Read the model definition and answer for the solid it produces. Units are mm, in the model's axes. A direction names the side the tool comes from. Round coordinates to 2 decimals unless told otherwise and drop trailing zeros. Order: outer loops, then holes, each group sorted by start corner. A loop starts at its lowest first (then second) coordinate and runs counter-clockwise, first axis right, second up. Notation, with made-up numbers: (62, 19) - (70, 19) arc R13 cw to (70, 34) - close; hole circle Ø11 at (44.25, 77). An arc over 180 degrees is marked (long way). Answer as a JSON object with one key per item and string values. Group by question number.
Q1. A cutting plane is placed at D-D on y = 9.1. Determine the outline of the cut face in (x, z), and give its area (3 significant figures).
Q2. A cutting plane is placed at A-A on y = 16.8. Determine the outline of the cut face in (x, z), and give its area (3 significant figures).
Q3. Given pin 1 Ø6.5 at (y, z) = (15, 10.5) entering from -X; pin 2 Ø6 at (y, z) = (23.5, 17.5) entering from -X, each flat-ended and moving along its own axis, determine where each tip first touches the part or whether it passes through.
Q4. A cutting plane is placed at C-C on x = 5. Determine the outline of the cut face in (y, z).
Q5. The mould has two halves that part along X. Classify faces 3 (the flat face through (0, 1, 12)), 4 (the cylindrical face through (18.71, 1.27, 11.07)), 5 (the cylindrical face through (27.56, 23.28, 4.82)): pulls with the +X half, pulls with the -X half, needs draft (parallel to the pull), parting line crosses it, or undercut.
Q6. A tool of negligible diameter and unlimited length cuts with its end or side. For faces 1 (the cylindrical face through (27.56, 8.34, 20.94)), 2 (the flat face through (26.086, 9, 9)), from which of +Z, -Z, +X, -X, +Y, -Y can it reach the whole face along a straight path? Write none if from no direction.
Q7. A cutting plane is placed at B-B on z = 12.25. Determine the outline of the cut face in (x, y), and give its area (3 significant figures).
Q8. Consider line 1 (X direction, y = 19.75, z = 23.25); line 2 (Z direction, x = 5, y = 0.85); line 3 (Y direction, x = 5.25, z = 7.75). Determine where each line is inside the solid, lowest interval first.
```python
from build123d import *

# Parameters (mm, degrees)
SKETCH1_W               = 2.914347554
SKETCH1_H               = 25
SKETCH1_W_2             = 29
SKETCH1_H_2             = 2.5
BOSS_EXTRUDE1_DEPTH     = 24.5
SKETCH2_R               = 1.25
CUT_EXTRUDE1_DEPTH      = 30
SKETCH3_R               = 1.75
CUT_EXTRUDE2_DEPTH      = 26
CUT_EXTRUDE2_DEPTH_BACK = 3.5
SKETCH4_R               = 8.25
CUT_EXTRUDE3_DEPTH      = 27.085652446
CUT_EXTRUDE3_DEPTH_BACK = 3.914347554
SKETCH5_W               = 2.914347554
SKETCH5_H               = 0.55
CUT_EXTRUDE4_DEPTH      = 1
CUT_EXTRUDE4_DEPTH_BACK = 25.5
CHAMFER1_SIZE           = 3


with BuildPart() as part:
    # Sketch1 → Boss-Extrude1 (new body)
    with BuildSketch(Plane.XY):
        with Locations((27.542826223, 15)):
            Rectangle(SKETCH1_W, SKETCH1_H)
        with Locations((14.5, 1.25)):
            Rectangle(SKETCH1_W_2, SKETCH1_H_2)
    extrude(amount=BOSS_EXTRUDE1_DEPTH)

    # Sketch2 → Cut-Extrude1 (cut, through all)
    with BuildSketch(Plane(origin=(29, 0, 0), x_dir=(0, 0, -1), z_dir=(1, 0, 0))):
        with Locations((-19.95, 24.5)):
            Circle(SKETCH2_R)
        with Locations((-4.55, 24.5)):
            Circle(SKETCH2_R)
        with Locations((-4.55, 9.1)):
            Circle(SKETCH2_R)
        with Locations((-19.95, 9.1)):
            Circle(SKETCH2_R)
    extrude(amount=-CUT_EXTRUDE1_DEPTH, mode=Mode.SUBTRACT)

    # Sketch3 → Cut-Extrude2 (cut, two sides)
    with BuildSketch(Plane(origin=(0, 2.5, 0), x_dir=(1, 0, 0), z_dir=(0, 1, 0))) as cut_extrude2_sk:
        with Locations((5, -12.25)):
            Circle(SKETCH3_R)
        with Locations((20, -12.25)):
            Circle(SKETCH3_R)
    extrude(amount=CUT_EXTRUDE2_DEPTH, mode=Mode.SUBTRACT)
    extrude(cut_extrude2_sk.sketch, amount=-CUT_EXTRUDE2_DEPTH_BACK, mode=Mode.SUBTRACT)

    # Sketch4 → Cut-Extrude3 (cut, two sides)
    with BuildSketch(Plane.ZY.offset(-26.085652446)) as cut_extrude3_sk:
        with Locations((12.25, 16.8)):
            Circle(SKETCH4_R)
    extrude(amount=CUT_EXTRUDE3_DEPTH, mode=Mode.SUBTRACT)
    extrude(cut_extrude3_sk.sketch, amount=-CUT_EXTRUDE3_DEPTH_BACK, mode=Mode.SUBTRACT)

    # Sketch5 → Cut-Extrude4 (cut, two sides)
    with BuildSketch(Plane.XY.offset(24.5)) as cut_extrude4_sk:
        with Locations((27.542826223, 27.225)):
            Rectangle(SKETCH5_W, SKETCH5_H)
    extrude(amount=CUT_EXTRUDE4_DEPTH, mode=Mode.SUBTRACT)
    extrude(cut_extrude4_sk.sketch, amount=-CUT_EXTRUDE4_DEPTH_BACK, mode=Mode.SUBTRACT)

    # Chamfer1
    chamfer1_edges = [part.edges().sort_by_distance(p)[0] for p in [
        (26.085652446, 2.5, 12.25),
    ]]
    chamfer(chamfer1_edges, length=CHAMFER1_SIZE)


solid = part.part
```
Result set:
{
 "1": {"outline": "(26.09, 0) - (29, 0) - (29, 3.3) - (26.09, 3.3) - close; (26.09, 5.8) - (29, 5.8) - (29, 9.29) - (26.09, 9.29) - close; (26.09, 15.21) - (29, 15.21) - (29, 18.7) - (26.09, 18.7) - close; (26.09, 21.2) - (29, 21.2) - (29, 24.5) - (26.09, 24.5) - close", "area": "39.6 mm²"},
 "2": {"outline": "(26.09, 0) - (29, 0) - (29, 4) - (26.09, 4) - close; (26.09, 20.5) - (29, 20.5) - (29, 24.5) - (26.09, 24.5) - close", "area": "23.3 mm²"},
 "3": {"pin 1": "passes through", "pin 2": "stops at x = 26.09"},
 "4": {"outline": "(0, 0) - (2.5, 0) - (2.5, 10.5) - (0, 10.5) - close; (0, 14) - (2.5, 14) - (2.5, 24.5) - (0, 24.5) - close"},
 "5": {"face 3": "pulls with the -X half", "face 4": "undercut", "face 5": "needs draft"},
 "6": {"face 1": "+X, -X", "face 2": "+Z, -Z, -X, +Y"},
 "7": {"outline": "(0, 0) - (3.25, 0) - (3.25, 2.5) - (0, 2.5) - close; (6.75, 0) - (18.25, 0) - (18.25, 2.5) - (6.75, 2.5) - close; (21.75, 0) - (29, 0) - (29, 8.55) - (26.09, 8.55) - (26.09, 5.5) - (23.09, 2.5) - (21.75, 2.5) - close; (26.09, 25.05) - (29, 25.05) - (29, 26.95) - (26.09, 26.95) - close", "area": "82.7 mm²"},
 "8": {"line 1": "x = 26.09 to 29", "line 2": "z = 0 to 10.5, 14 to 24.5", "line 3": "y = 0 to 2.5"}
}
